The listing builds one solid part. Answer for the finished solid, in the listing's coordinates (mm). Give positions to 0.01 mm unless a question says otherwise; leave off trailing zeros. Write each loop counter-clockwise with the first axis right and the second up, starting at its lowest first coordinate (ties: lowest second). Pieces come first, ordered by that corner, then holes. Notation, with made-up numbers: (84, 28) - (126, 28) arc R4 ccw to (126, 34) - close; hole circle Ø1 at (88.25, 23.5). An arc over 180 degrees is marked (long way). Use a Markdown table: item, result. Add a question column.
from build123d import *

# Parameters (mm, degrees)
ESQUISSE1_W             = 680
ESQUISSE1_H             = 210
BOSS_EXTRU_1_DEPTH      = 10
ESQUISSE2_W             = 80
ESQUISSE2_H             = 24
ENL_V_MAT_EXTRU_1_DEPTH = 11
ESQUISSE3_R             = 5
ENL_V_MAT_EXTRU_2_DEPTH = 11


with BuildPart() as part:
    # Esquisse1 → Boss.-Extru.1 (new body)
    with BuildSketch(Plane.XY):
        Rectangle(ESQUISSE1_W, ESQUISSE1_H)
    extrude(amount=BOSS_EXTRU_1_DEPTH)

    # Esquisse2 → Enlèv. mat.-Extru.1 (cut, through all)
    with BuildSketch(Plane.XY.offset(10)):
        with Locations((-300, -93)):
            Rectangle(ESQUISSE2_W, ESQUISSE2_H)
        with Locations((300, -93)):
            Rectangle(ESQUISSE2_W, ESQUISSE2_H)
    extrude(amount=-ENL_V_MAT_EXTRU_1_DEPTH, mode=Mode.SUBTRACT)

    # Esquisse3 → Enlèv. mat.-Extru.2 (cut, through all)
    with BuildSketch(Plane.XY.offset(10)):
        with Locations((-320, -46)):
            Circle(ESQUISSE3_R)
    extrude(amount=-ENL_V_MAT_EXTRU_2_DEPTH, mode=Mode.SUBTRACT)


solid = part.part
1. Given P1, Ø3, axis at y = -90.5, z = 5, coming from the +X side; P2, Ø5, axis at y = -93.5, z = 5.5, coming from the -X side; P3, Ø5, axis at x = -292.5, z = 4, coming from the -Y side; P4, Ø8, axis at x = -320, y = -46, coming from the +Z side, each flat-ended and moving along its own axis, determine where each tip first touches the part or whether it passes through.
2. The part is cut by section B-B (x = 291.5). Give the vertices of the cut face in (y, z), and give its area (3 significant figures).
3. Consider L1, parallel to Y at x = -320, z = 7.5; L2, parallel to X at y = -84, z = 6.5. Determine where each line is inside the solid, lowest interval first. Write a range as [from, to].
4. The part is cut by section A-A (z = 5.25). Give the vertices of the cut face in (x, y), and give its area (3 significant figures).
Check values:
| question | item | result |
|---|---|---|
| 1 | P1 | stops at x = 260 |
| 1 | P2 | stops at x = -260 |
| 1 | P3 | stops at y = -81 |
| 1 | P4 | passes through |
| 2 | outline | (-81, 0) - (105, 0) - (105, 10) - (-81, 10) - close |
| 2 | area | 1,860 mm2 |
| 3 | L1 | y = [-81, -51], [-41, 105] |
| 3 | L2 | x = [-260, 260] |
| 4 | outline | (-340, -81) - (-260, -81) - (-260, -105) - (260, -105) - (260, -81) - (340, -81) - (340, 105) - (-340, 105) - close; hole circle Ø10 at (-320, -46) |
| 4 | area | 139,000 mm2 |
